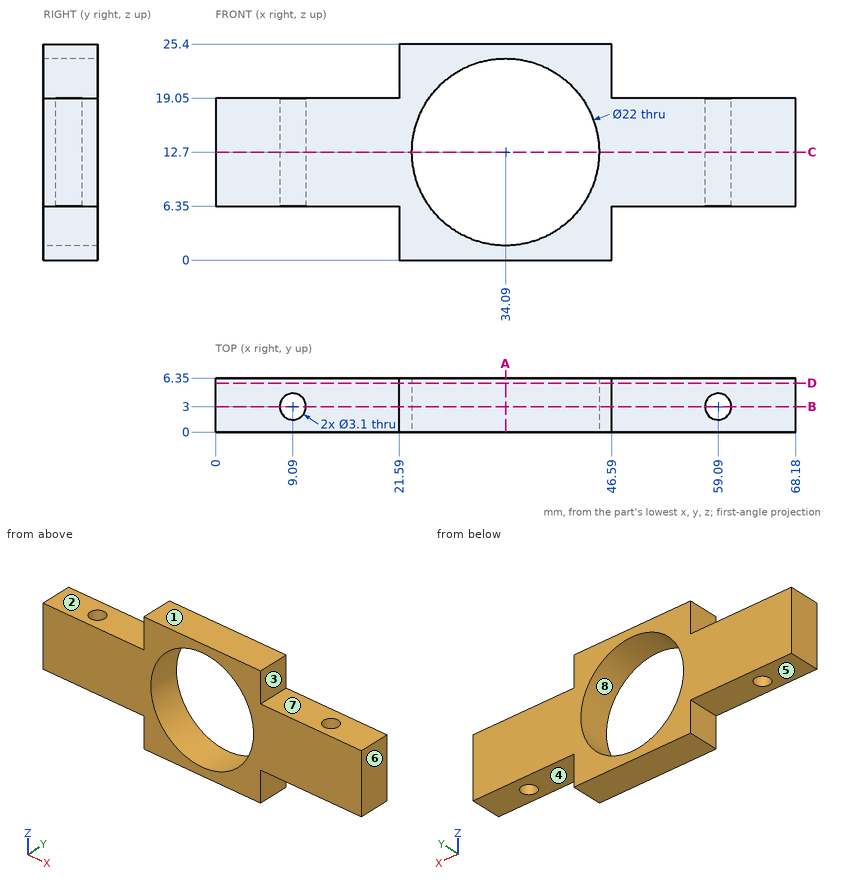
The figure shows three views and two pictorial views of one solid part (mm, origin at its lowest corner). Answer the questions. A direction names the side the tool comes from. Give positions to 0.01 mm unless a question says otherwise; leave off trailing zeros. Loops run counter-clockwise (first coordinate to the right, second up) from the corner with the lowest first, then second, coordinate; pieces in that order, holes last. Notation, with made-up numbers: (66, -3.5) - (74, -3.5) arc R21 cw to (74, 0.5) - close; hole circle Ø3 at (89, 44.5). An arc over 180 degrees is marked (long way). Answer in a Markdown table with one row per item.
(1) Section D-D (y = 5.75) is taken. Give the vertices of the cut face in (x, z).
Results list:
| item | result |
|---|---|
| outline | (0, 6.35) - (21.59, 6.35) - (21.59, 0) - (46.59, 0) - (46.59, 6.35) - (68.18, 6.35) - (68.18, 19.05) - (46.59, 19.05) - (46.59, 25.4) - (21.59, 25.4) - (21.59, 19.05) - (0, 19.05) - close; hole circle Ø22 at (34.09, 12.7) |
(2) Flat-ended cylindrical pins translate along their axes: pin 1 Ø1.9 at (x, y) = (15, 2.5) entering from +Z; pin 2 Ø3 at (x, z) = (48.5, 4.5) entering from -Y; pin 3 Ø1.9 at (x, y) = (62.5, 2.5) entering from -Z. Find the tip coordinate at first contact, or state that the pin passes through.
Results list:
| item | result |
|---|---|
| pin 1 | stops at z = 19.05 |
| pin 2 | passes through |
| pin 3 | stops at z = 6.35 |
(3) Section C-C (z = 12.7) is taken. Give the vertices of the cut face in (x, y), and give its area (3 significant figures).
Results list:
| item | result |
|---|---|
| outline | (0, 0) - (23.09, 0) - (23.09, 6.35) - (0, 6.35) - close; (45.09, 0) - (68.18, 0) - (68.18, 6.35) - (45.09, 6.35) - close; hole circle Ø3.1 at (9.09, 3); hole circle Ø3.1 at (59.09, 3) |
| area | 278 mm² |
(4) Section B-B (y = 3) is taken. Give the vertices of the cut face in (x, z).
Results list:
| item | result |
|---|---|
| outline | (0, 6.35) - (7.54, 6.35) - (7.54, 19.05) - (0, 19.05) - close; (10.64, 6.35) - (21.59, 6.35) - (21.59, 0) - (46.59, 0) - (46.59, 6.35) - (57.54, 6.35) - (57.54, 19.05) - (46.59, 19.05) - (46.59, 25.4) - (21.59, 25.4) - (21.59, 19.05) - (10.64, 19.05) - close; (60.64, 6.35) - (68.18, 6.35) - (68.18, 19.05) - (60.64, 19.05) - close; hole circle Ø22 at (34.09, 12.7) |
(5) Section A-A (x = 34.09) is taken. Give the vertices of the cut face in (y, z).
Results list:
| item | result |
|---|---|
| outline | (0, 0) - (6.35, 0) - (6.35, 1.7) - (0, 1.7) - close; (0, 23.7) - (6.35, 23.7) - (6.35, 25.4) - (0, 25.4) - close |
(6) For a pull along Z with two mould halves and no side action, classify the marked faces 6, 7 and 8 as pulls with the +Z half, pulls with the -Z half, needs draft (parallel to the pull), parting line crosses it, or undercut.
Results list:
| item | result |
|---|---|
| face 6 | needs draft |
| face 7 | pulls with the +Z half |
| face 8 | undercut |
(7) Consider L1, parallel to X at y = 3, z = 12.25; L2, parallel to X at y = 3, z = 9.5; L3, parallel to Y at x = 9.09, z = 10. Determine where each line is inside the solid, lowest interval first. Write a range as [from, to].
Results list:
| item | result |
|---|---|
| L1 | x = [0, 7.54], [10.64, 23.1], [45.08, 57.54], [60.64, 68.18] |
| L2 | x = [0, 7.54], [10.64, 23.57], [44.61, 57.54], [60.64, 68.18] |
| L3 | y = [0, 1.45], [4.55, 6.35] |
(8) A tool of negligible diameter and unlimited length cuts with its end or side. For the marked faces 1, 2, 3, 4 and 5, from which of +Z, -Z, +X, -X, +Y, -Y can it reach the whole face along a straight path? Write none if from no direction.
Results list:
| item | result |
|---|---|
| face 1 | +Z, +X, -X, +Y, -Y |
| face 2 | +Z, -X, +Y, -Y |
| face 3 | +Z, +X, +Y, -Y |
| face 4 | -Z, +X, +Y, -Y |
| face 5 | -Z, -X, +Y, -Y |
